For this review, take the finished solid that the model builds, in its own axes (mm). Give positions to 0.01 mm unless a question says otherwise; leave off trailing zeros. Loops run counter-clockwise (first coordinate to the right, second up) from the corner with the lowest first, then second, coordinate; pieces in that order, holes last.
```python
from build123d import *

# Parameters (mm, degrees)
F0_R     = 2.25
F0_R_2   = 1.75
F0_R_3   = 18
F0_R_4   = 4.1
F1_DEPTH = 3


with BuildPart() as f1:
    # F0 (on Front) → F1 (new body)
    with BuildSketch(Plane.XZ):
        with BuildLine():
            ThreePointArc((110, 32.5), (108.535534, 36.035534), (105, 37.5))
            Line((105, 37.5), (-105, 37.5))
            ThreePointArc((-105, 37.5), (-108.535534, 36.035534), (-110, 32.5))
            Line((-110, 32.5), (-110, -32.5))
            ThreePointArc((-110, -32.5), (-108.535534, -36.035534), (-105, -37.5))
            Line((-105, -37.5), (105, -37.5))
            ThreePointArc((105, -37.5), (108.535534, -36.035534), (110, -32.5))
            Line((110, -32.5), (110, 32.5))
        make_face()
        with Locations((-102, -29.5)):
            Circle(F0_R, mode=Mode.SUBTRACT)
        with BuildLine():
            ThreePointArc((-72.089674, 5.7), (-75, -6.4), (-77.910326, 5.7))
            Line((-77.910326, 5.7), (-72.089674, 5.7))
        make_face(mode=Mode.SUBTRACT)
        with Locations((-17, -17)):
            Circle(F0_R_2, mode=Mode.SUBTRACT)
        with Locations((0, -29.5)):
            Circle(F0_R, mode=Mode.SUBTRACT)
        with Locations((102, -29.5)):
            Circle(F0_R, mode=Mode.SUBTRACT)
        with Locations((17, -17)):
            Circle(F0_R_2, mode=Mode.SUBTRACT)
        with Locations((-17, 17)):
            Circle(F0_R_2, mode=Mode.SUBTRACT)
        with Locations((-102, 29.5)):
            Circle(F0_R, mode=Mode.SUBTRACT)
        Circle(F0_R_3, mode=Mode.SUBTRACT)
        with Locations((17, 17)):
            Circle(F0_R_2, mode=Mode.SUBTRACT)
        with Locations((75, 0)):
            Circle(F0_R_4, mode=Mode.SUBTRACT)
        with Locations((0, 29.5)):
            Circle(F0_R, mode=Mode.SUBTRACT)
        with Locations((102, 29.5)):
            Circle(F0_R, mode=Mode.SUBTRACT)
    extrude(amount=F1_DEPTH)


solid = f1.part
```
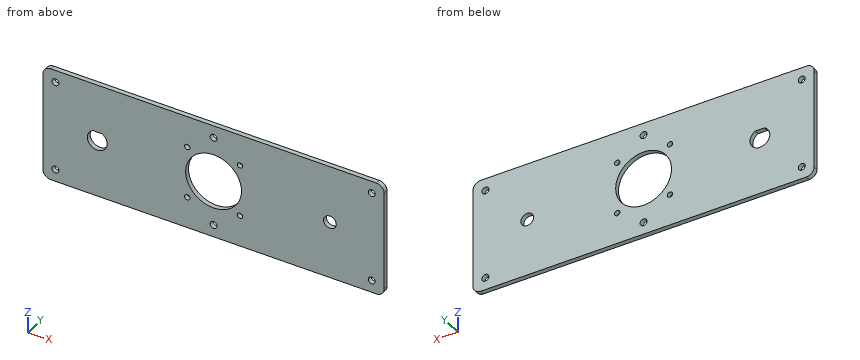
Item 1: For L1, parallel to Z at x = 102, y = -0.65; L2, parallel to X at y = -2.4, z = -16; L3, parallel to X at y = -0.4, z = 3.5, list the stretches that pass through material, from the lowest coordinate up.
Answer:
L1: z = -37.5 to -31.75, -27.25 to 27.25, 31.75 to 37.5
L2: x = -110 to -18.44, -15.56 to -8.25, 8.25 to 15.56, 18.44 to 110
L3: x = -110 to -80.36, -69.64 to -17.66, 17.66 to 72.86, 77.14 to 110
Item 2: Take a section at D-D on y = -1.2. State how many separate pieces and enclosed holes the cut face has, and give its area (3 significant figures).
Answer:
separate pieces: 1
enclosed holes: 13
area: 15,100 mm2
Item 3: Take a section at A-A on x = -102. Give the boundary of the cut face in (y, z).
Answer:
outline: (-3, -37.5) - (0, -37.5) - (0, -31.75) - (-3, -31.75) - close; (-3, -27.25) - (0, -27.25) - (0, 27.25) - (-3, 27.25) - close; (-3, 31.75) - (0, 31.75) - (0, 37.5) - (-3, 37.5) - close
Item 4: Take a section at B-B on z = 0. Give the boundary of the cut face in (x, y).
Answer:
outline: (-110, -3) - (-81.4, -3) - (-81.4, 0) - (-110, 0) - close; (-68.6, -3) - (-18, -3) - (-18, 0) - (-68.6, 0) - close; (18, -3) - (70.9, -3) - (70.9, 0) - (18, 0) - close; (79.1, -3) - (110, -3) - (110, 0) - (79.1, 0) - close
Item 5: Take a section at C-C on x = 75. Give the boundary of the cut face in (y, z), and give its area (3 significant figures).
Answer:
outline: (-3, -37.5) - (0, -37.5) - (0, -4.1) - (-3, -4.1) - close; (-3, 4.1) - (0, 4.1) - (0, 37.5) - (-3, 37.5) - close
area: 200 mm2
